Geometry: final body of the model. Coordinates: model frame, mm. Face numbers are marked on the shaded views. A direction names the side the tool comes from. Coordinates: 2 decimals unless noted, no trailing zeros. Write each loop counter-clockwise with the first axis right and the second up, starting at its lowest first coordinate (ties: lowest second). Pieces come first, ordered by that corner, then holes. Notation, with made-up numbers: (79, 8) -> (127, 8) arc R18 ccw to (127, 41) -> close; hole circle Ø5 at (36.25, 59). An arc over 180 degrees is marked (long way). One line per item, written item: value.
```python
from build123d import *

# Parameters (mm, degrees)
SKETCH1_R           = 5.5
SKETCH1_R_2         = 0.5
BOSS_EXTRUDE1_DEPTH = 6
SKETCH2_R           = 5.5
BOSS_EXTRUDE2_DEPTH = 1
SKETCH3_R           = 0.5
CUT_EXTRUDE1_DEPTH  = 7
SKETCH4_W           = 5
SKETCH4_H           = 5
BOSS_EXTRUDE3_DEPTH = 0.1
SKETCH5_OUTSIDE_W   = 16.342
SKETCH5_OUTSIDE_H   = 16.342
SKETCH5_OUTSIDE_W_2 = 5
SKETCH5_OUTSIDE_H_2 = 5
CUT_EXTRUDE2_DEPTH  = 3.6


with BuildPart() as part:
    # Sketch1 → Boss-Extrude1 (new body)
    with BuildSketch(Plane(origin=(0, 0, 0), x_dir=(0, 0, -1), z_dir=(1, 0, 0))):
        Circle(SKETCH1_R)
        with Locations((0, 4)):
            Circle(SKETCH1_R_2, mode=Mode.SUBTRACT)
        with Locations((4, 0)):
            Circle(SKETCH1_R_2, mode=Mode.SUBTRACT)
        with Locations((0, -4)):
            Circle(SKETCH1_R_2, mode=Mode.SUBTRACT)
        with Locations((-4, 0)):
            Circle(SKETCH1_R_2, mode=Mode.SUBTRACT)
        with BuildLine():
            Line((-1.321221026, 1.6), (1.321221026, 1.6))
            ThreePointArc((1.321221026, 1.6), (0, -2.075), (-1.321221026, 1.6))
        make_face(mode=Mode.SUBTRACT)
    extrude(amount=BOSS_EXTRUDE1_DEPTH)

    # Sketch2 → Boss-Extrude2 (add)
    with BuildSketch(Plane(origin=(6, 0, 0), x_dir=(0, 0, -1), z_dir=(1, 0, 0))):
        Circle(SKETCH2_R)
    extrude(amount=-BOSS_EXTRUDE2_DEPTH)

    # Sketch3 → Cut-Extrude1 (cut, through all)
    with BuildSketch(Plane.ZY):
        with Locations((0, 4)):
            Circle(SKETCH3_R)
        with Locations((4, 0)):
            Circle(SKETCH3_R)
        with Locations((0, -4)):
            Circle(SKETCH3_R)
        with Locations((-4, 0)):
            Circle(SKETCH3_R)
    extrude(amount=-CUT_EXTRUDE1_DEPTH, mode=Mode.SUBTRACT)

    # Sketch4 → Boss-Extrude3 (add)
    with BuildSketch(Plane(origin=(6, 0, 0), x_dir=(0, 0, -1), z_dir=(1, 0, 0))):
        Rectangle(SKETCH4_W, SKETCH4_H)
    extrude(amount=BOSS_EXTRUDE3_DEPTH)

    # Sketch5 outside → Cut-Extrude2 (cut)
    with BuildSketch(Plane(origin=(6, 0, 0), x_dir=(0, 0, -1), z_dir=(1, 0, 0))):
        Rectangle(SKETCH5_OUTSIDE_W, SKETCH5_OUTSIDE_H)
        Rectangle(SKETCH5_OUTSIDE_W_2, SKETCH5_OUTSIDE_H_2, mode=Mode.SUBTRACT)
    extrude(amount=-CUT_EXTRUDE2_DEPTH, mode=Mode.SUBTRACT)


solid = part.part
```
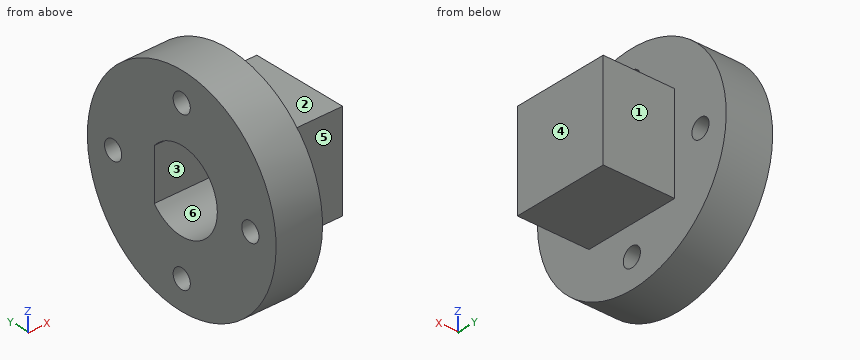
(1) First-contact query: pin 1 (1 mm diameter, centred on x = 2.5, y = 0, fed in from +Z); pin 2 (1.8 mm diameter, centred on x = 3.5, y = 0.5, fed in from +Z); pin 3 (3 mm diameter, centred on x = 4.5, z = -0.5, fed in from +Y); pin 4 (1 mm diameter, centred on x = 3.5, z = -1, fed in from -Y). Flat tips, straight axial feed; report the tip coordinate or a pass-through.
Responses:
pin 1: stops at z = 5.5
pin 2: stops at z = 2.5
pin 3: stops at y = 2.5
pin 4: stops at y = -2.5
(2) Section B-B (x = 0.75). Return the cut outline in (y, z) (3 decimals), then the cut area to 3 significant figures.
Responses:
outline: circle Ø11 at (0, 0); hole circle Ø1 at (-4, 0); hole circle Ø1 at (0, -4); hole circle Ø1 at (0, 4); hole (1.6, -1.321) -> (1.6, 1.321) arc R2.075 ccw (long way) to start; hole circle Ø1 at (4, 0)
area: 79.2 mm2
(3) Line query: line 1 (Z direction, x = 0.5, y = 0) (3 decimals); line 2 (Z direction, x = 2.75, y = 0) (3 decimals); line 3 (Z direction, x = 1.4, y = 4). Output: solid intervals per line, ascending. Write a range as [from, to].
Responses:
line 1: z = [-5.5, -4.5], [-3.5, -2.075], [2.075, 3.5], [4.5, 5.5]
line 2: z = [-2.5, -2.075], [2.075, 2.5]
line 3: z = [-3.77, -0.5], [0.5, 3.77]
(4) Section C-C (z = 4). Return the cut outline in (x, y).
Responses:
outline: (0, -3.77) -> (2.4, -3.77) -> (2.4, -0.5) -> (0, -0.5) -> close; (0, 0.5) -> (2.4, 0.5) -> (2.4, 3.77) -> (0, 3.77) -> close
(5) Section A-A (y = 0). Return the cut outline in (x, z) (3 decimals), then the cut area to 4 significant figures.
Responses:
outline: (0, -5.5) -> (2.4, -5.5) -> (2.4, -4.5) -> (0, -4.5) -> close; (0, -3.5) -> (2.4, -3.5) -> (2.4, -2.5) -> (6.1, -2.5) -> (6.1, 2.5) -> (2.4, 2.5) -> (2.4, 3.5) -> (0, 3.5) -> (0, 2.075) -> (5, 2.075) -> (5, -2.075) -> (0, -2.075) -> close; (0, 4.5) -> (2.4, 4.5) -> (2.4, 5.5) -> (0, 5.5) -> close
area: 19.35 mm2
(6) Pull-direction query (Y, two-part tool) for the marked faces 4, 5 and 6; classes: released by +Y, released by -Y, zero draft, split by the parting line, or undercut.
Responses:
face 4: zero draft
face 5: released by -Y
face 6: undercut
(7) Reachability of the marked faces 1, 2 and 3 from +Z, -Z, +X, -X, +Y, -Y: full face, straight path, thin tool, end or side. Return the list, or none.
Responses:
face 1: +Z, -Z, +X, +Y
face 2: +Z, +X, +Y, -Y
face 3: -X
